The listing builds one solid part. Answer for the finished solid, in the listing's coordinates (mm). Give positions to 0.01 mm unless a question says otherwise; leave off trailing zeros. Order: outer loops, then holes, each group sorted by start corner. A loop starts at its lowest first (then second) coordinate and runs counter-clockwise, first axis right, second up. Notation, with made-up numbers: (-10, 1) - (22, 1) arc R34 cw to (22, 39) - close; hole circle Ø7 at (67.25, 51). An arc over 180 degrees is marked (long way). Use a Markdown table: item, result. Add a question column.
1) Straight lines are drawn through the part: line 1 (Y direction, x = -36.5, z = 7.75); line 2 (Y direction, x = 32.5, z = 2); line 3 (X direction, y = -44.5, z = 11.5). For each, find the intervals that lie inside material, in ascending order.
2) A flat-ended cylindrical pin translates along its axis: pin 1 (8 mm diameter, centred on x = 36.5, y = 43.5, fed in from +Z). Find the tip coordinate at first contact, or state that the pin passes through.
3) The mould has two halves that part along Y. Classify faces 1 (the face through (43.243, 43.797, 6.902)), 2 (the face through (46.5, -1, 7)), 3 (the face through (-1, -53.5, 7)): released by +Y, released by -Y, zero draft, split by the parting line, or undercut.
4) Find section A-A, the plane z = 12.5. Determine the outline of the cut face in (x, y).
from build123d import *

# Parameters (mm, degrees)
SKICA1_W                 = 93
SKICA1_H                 = 107
P_IDAT_VYSUNUT_M1_DEPTH  = 14
SKICA2_R                 = 6.75
ODEBRAT_VYSUNUT_M1_DEPTH = 15
SKICA4_W                 = 75
SKICA4_H                 = 53
ODEBRAT_VYSUNUT_M2_DEPTH = 0.0001


with BuildPart() as part:
    # Skica1 → Přidat vysunutím1 (new body)
    with BuildSketch(Plane.XY):
        Rectangle(SKICA1_W, SKICA1_H)
    extrude(amount=P_IDAT_VYSUNUT_M1_DEPTH)

    # Skica2 → Odebrat vysunutím1 (cut, through all)
    with BuildSketch(Plane(origin=(0, 0, 0), x_dir=(-1, 0, 0), z_dir=(0, 0, -1))):
        with Locations((-36.5, 43.5)):
            Circle(SKICA2_R)
        with Locations((36.5, 43.5)):
            Circle(SKICA2_R)
        with Locations((36.5, -43.5)):
            Circle(SKICA2_R)
        with Locations((-36.5, -43.5)):
            Circle(SKICA2_R)
    extrude(amount=-ODEBRAT_VYSUNUT_M1_DEPTH, mode=Mode.SUBTRACT)

    # Skica4 → Odebrat vysunutím2 (cut)
    with BuildSketch(Plane(origin=(0, 0, 0), x_dir=(-1, 0, 0), z_dir=(0, 0, -1))):
        Rectangle(SKICA4_W, SKICA4_H)
    extrude(amount=-ODEBRAT_VYSUNUT_M2_DEPTH, mode=Mode.SUBTRACT)


solid = part.part
The answers:
| question | item | result |
|---|---|---|
| 1 | line 1 | -53.5 to -50.25, -36.75 to 36.75, 50.25 to 53.5 |
| 1 | line 2 | -53.5 to -48.94, -38.06 to 38.06, 48.94 to 53.5 |
| 1 | line 3 | -46.5 to -43.18, -29.82 to 29.82, 43.18 to 46.5 |
| 2 | pin 1 | through |
| 3 | face 1 | undercut |
| 3 | face 2 | zero draft |
| 3 | face 3 | released by -Y |
| 4 | outline | (-46.5, -53.5) - (46.5, -53.5) - (46.5, 53.5) - (-46.5, 53.5) - close; hole circle Ø13.5 at (-36.5, -43.5); hole circle Ø13.5 at (-36.5, 43.5); hole circle Ø13.5 at (36.5, -43.5); hole circle Ø13.5 at (36.5, 43.5) |
